Check sheet for the modelled part. Datum: model origin and axes. Units: mm. Face numbers are marked on the shaded views. A direction names the side the tool comes from. Round coordinates to 2 decimals unless told otherwise and drop trailing zeros. Loops run counter-clockwise (first coordinate to the right, second up) from the corner with the lowest first, then second, coordinate; pieces in that order, holes last. Notation, with made-up numbers: (-40, -5.5) - (-29, -5.5) arc R30 cw to (-29, 30.5) - close; hole circle Ø10 at (36.5, 27.5). An arc over 180 degrees is marked (long way). Answer in a Markdown table with one row per item. Add a question column.
(1) Cross-section at A-A on y = 24. Enter the section's corners in (x, z) (3 decimals).
(2) Cross-section at B-B on z = -1. Enter the section's corners in (x, y) (3 decimals), then the cut area to 3 significant figures.
(3) Access from +Z, -Z, +X, -X, +Y, -Y to the whole of each face (thin tool, end or side, straight path). Record for the marked faces 1, 2, 3, 4 and 5.
(4) Gauge pin test, flat ends, axial feed: pin 1 (3 mm diameter, centred on x = -2, z = 36.5, fed in from +Y); pin 2 (12 mm diameter, centred on x = 5.5, y = 20, fed in from +Z) (3 decimals); pin 3 (1.5 mm diameter, centred on x = 73, z = 45.5, fed in from +Y). Record the tip position at first contact, or that the pin passes through.
(5) Thickness scan on line 1 along Z through (x, y) = (68.5, -46); line 2 along Y through (x, z) = (-18, 32.5); line 3 along Y through (x, z) = (63, 43). Record the ranges inside material, lowest first.
(6) Mould release check, pull along Z, two halves, no side actions. Record for the marked faces 6, 7 and 8: +Z half, -Z half, draft (parallel to the pull), parting line (faces both ways), or undercut.
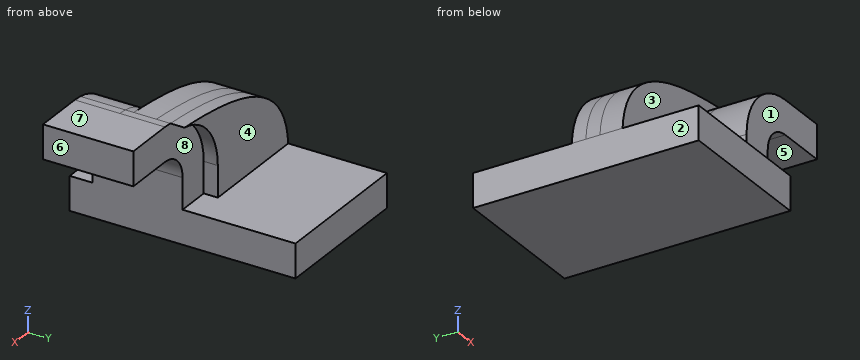
from build123d import *

# Parameters (mm, degrees)
F1_DEPTH  = 63.5
F2_DEPTH  = 25.4
F3_DEPTH  = 25.4
F3_FACE_W = 50.8
F3_FACE_H = 19.05
F4_DEPTH  = 25.4
F5_DEPTH  = 7.9375
F6_DEPTH  = 12.7


with BuildPart() as f1:
    # F0 (on Front) → F1 (new body, symmetric)
    with BuildSketch(Plane.XZ):
        Polygon((22.225, 9.525), (-41.275, 9.525), (-41.275, -9.525), (41.275, -9.525), (41.275, 9.525), align=None)
    extrude(amount=F1_DEPTH, both=True)

    # F0 (on Front) → F2 (join)
    with BuildSketch(Plane.XZ):
        with BuildLine():
            Line((22.225, 27.0002), (22.225, 9.525))
            Line((22.225, 9.525), (41.275, 9.525))
            Line((41.275, 9.525), (41.275, 27.0002))
            ThreePointArc((41.275, 27.0002), (45.92468, 38.22552), (57.15, 42.8752))
            Line((57.15, 42.8752), (60.325, 42.8752))
            Line((60.325, 42.8752), (60.325, 61.9252))
            Line((60.325, 61.9252), (57.15, 61.9252))
            add(Edge.make_bspline(
                [(52.222263, 61.575813), (53.87533, 61.698715), (55.518942, 61.814596), (57.15, 61.9252)],
                knots=[107.296838, 107.296838, 107.296838, 107.296838, 111.504536, 111.504536, 111.504536, 111.504536], degree=3))
            ThreePointArc((52.222263, 61.575813), (30.769545, 49.887472), (22.225, 27.0002))
        make_face()
    extrude(amount=F2_DEPTH)

    # F2_face (on face) → F3 (join, symmetric)
    with BuildSketch(Plane(origin=(38.743879, -25.4, 36.959126), x_dir=(1, 0, 0), z_dir=(0, -1, 0))):
        with BuildLine():
            ThreePointArc((13.478383, 24.616687), (-7.974335, 12.928345), (-16.518879, -9.958926))
            Line((-16.518879, -9.958926), (-16.518879, -27.434126))
            Line((-16.518879, -27.434126), (2.531121, -27.434126))
            Line((2.531121, -27.434126), (2.531121, -9.958926))
            ThreePointArc((2.531121, -9.958926), (7.180801, 1.266394), (18.406121, 5.916074))
            Line((18.406121, 5.916074), (21.581121, 5.916074))
            Line((21.581121, 5.916074), (21.581121, 24.966074))
            Line((21.581121, 24.966074), (18.406121, 24.966074))
            add(Edge.make_bspline(
                [(13.478383, 24.616687), (15.131451, 24.739589), (16.775063, 24.855469), (18.406121, 24.966074)],
                knots=[107.296838, 107.296838, 107.296838, 107.296838, 111.504536, 111.504536, 111.504536, 111.504536], degree=3))
        make_face()
    extrude(amount=F3_DEPTH, both=True)

    # F3_face (on face) → F4 (join)
    with BuildSketch(Plane(origin=(60.325, -25.4, 52.4002), x_dir=(0, 1, 0), z_dir=(1, 0, 0))):
        Rectangle(F3_FACE_W, F3_FACE_H)
    extrude(amount=F4_DEPTH)

    # F0 (on Front) → F5 (join, symmetric)
    with BuildSketch(Plane.XZ):
        with BuildLine():
            add(Edge.make_bspline(
                [(-41.275, 9.525), (-38.232598, 50.741845), (10.068833, 58.441796), (52.222263, 61.575813)],
                knots=[0, 0, 0, 0, 107.296838, 107.296838, 107.296838, 107.296838], degree=3))
            Line((-41.275, 9.525), (22.225, 9.525))
            Line((22.225, 9.525), (22.225, 27.0002))
            ThreePointArc((22.225, 27.0002), (30.769545, 49.887472), (52.222263, 61.575813))
        make_face()
    extrude(amount=F5_DEPTH, both=True)

    # F5_face (on face) → F6 (join, symmetric)
    with BuildSketch(Plane(origin=(-1.735733, -7.9375, 31.373848), x_dir=(1, 0, 0), z_dir=(0, -1, 0))):
        with BuildLine():
            add(Edge.make_bspline(
                [(-39.539267, -21.848848), (-36.496865, 19.367997), (11.804566, 27.067948), (53.957996, 30.201965)],
                knots=[0, 0, 0, 0, 107.296838, 107.296838, 107.296838, 107.296838], degree=3))
            Line((-39.539267, -21.848848), (23.960733, -21.848848))
            Line((23.960733, -21.848848), (23.960733, -4.373648))
            ThreePointArc((23.960733, -4.373648), (32.505278, 18.513623), (53.957996, 30.201965))
        make_face()
    extrude(amount=F6_DEPTH, both=True)


solid = f1.part
Answers:
| question | item | result |
|---|---|---|
| 1 | outline | (-41.275, -9.525) - (41.275, -9.525) - (41.275, 9.525) - (-41.275, 9.525) - close |
| 2 | outline | (-41.275, -63.5) - (41.275, -63.5) - (41.275, 63.5) - (-41.275, 63.5) - close |
| 2 | area | 10,500 mm^2 |
| 3 | face 1 | +Z, +X, -X, -Y |
| 3 | face 2 | +Z, -Z, -X, +Y, -Y |
| 3 | face 3 | +Z, -X, -Y |
| 3 | face 4 | +Z, +X, -X, +Y |
| 3 | face 5 | -Z, +X, +Y, -Y |
| 4 | pin 1 | stops at y = 7.94 |
| 4 | pin 2 | stops at z = 9.525 |
| 4 | pin 3 | stops at y = 0 |
| 5 | line 1 | z = 42.88 to 61.93 |
| 5 | line 2 | y = -20.64 to 7.94 |
| 5 | line 3 | y = -50.8 to 0 |
| 6 | face 6 | draft |
| 6 | face 7 | +Z half |
| 6 | face 8 | undercut |
